Here's how the part is built. I have some questions about the finished solid (model axes, mm). A direction names the side the tool comes from. Round coordinates to 2 decimals unless told otherwise and drop trailing zeros. Order: outer loops, then holes, each group sorted by start corner. A loop starts at its lowest first (then second) coordinate and runs counter-clockwise, first axis right, second up. Notation, with made-up numbers: (-21.5, 78) - (18.5, 78) arc R23 cw to (18.5, 106) - close; hole circle Ø6 at (66.25, 24). An arc over 180 degrees is marked (long way). Answer as a JSON object with one key per item and string values.
```python
from build123d import *

# Parameters (mm, degrees)
SKETCH_1_R          = 35
EXTRUDE_2_DEPTH     = 63.5
SKETCH_3_R          = 2
CUT_EXTRUDE_1_DEPTH = 20


with BuildPart() as part:
    # 草图1 → 凸台-拉伸2 (new body)
    with BuildSketch(Plane.XY):
        Circle(SKETCH_1_R)
    extrude(amount=EXTRUDE_2_DEPTH)

    # 草图3 → 切除-拉伸1 (cut)
    with BuildSketch(Plane.XY.offset(63.5)):
        with Locations((-23, 0)):
            Circle(SKETCH_3_R)
        with Locations((-11.5, 19.918584287)):
            Circle(SKETCH_3_R)
        with Locations((11.5, 19.918584287)):
            Circle(SKETCH_3_R)
        with Locations((23, 0)):
            Circle(SKETCH_3_R)
        with Locations((11.5, -19.918584287)):
            Circle(SKETCH_3_R)
        with Locations((-11.5, -19.918584287)):
            Circle(SKETCH_3_R)
    cut_extrude_1 = extrude(amount=-CUT_EXTRUDE_1_DEPTH, mode=Mode.SUBTRACT)

    # 镜向1: 切除-拉伸1 across plane
    add(cut_extrude_1.mirror(Plane.XY.offset(31.75)), mode=Mode.SUBTRACT)


solid = part.part
```
1. For faces 3 (the face through (-13.087, 18.702, 9.86)), 4 (the face through (-13.087, 18.702, 53.64)), 5 (the face through (0, 0, 63.5)), which set-ups out of +Z, -Z, +X, -X, +Y, -Y let a thin tool reach every point of the face, with its end or its side?
Responses:
{"face 3": "-Z", "face 4": "+Z", "face 5": "+Z, +X, -X, +Y, -Y"}
2. If I drill on L1, parallel to Y at x = -11, z = 48; L2, parallel to X at y = 19, z = 15; L3, parallel to Y at x = 11.5, z = 53, over which ranges is the centre line in solid material (lowest first)? Write a range as [from, to].
Responses:
{"L1": "[-33.23, -21.86], [-17.98, 17.98], [21.86, 33.23]", "L2": "[-29.39, -13.28], [-9.72, 9.72], [13.28, 29.39]", "L3": "[-33.06, -21.92], [-17.92, 17.92], [21.92, 33.06]"}
3. Thinking about a two-plate mould opening in Y: for faces 1 (the face through (9.913, 18.702, 9.86)), 2 (the face through (0, 0, 0)), which applies, pulls with the +Y half, pulls with the -Y half, needs draft (parallel to the pull), parting line crosses it, or undercut?
Responses:
{"face 1": "undercut", "face 2": "needs draft"}
4. Imagine slicing it at D-D (z = 38). List the corners of the cut face in (x, y) for me.
Responses:
{"outline": "circle Ø70 at (0, 0)"}
5. Imagine slicing it at B-B (z = 50.5). List the corners of the cut face in (x, y) for me, plus the area to 3 significant figures.
Responses:
{"outline": "circle Ø70 at (0, 0); hole circle Ø4 at (-23, 0); hole circle Ø4 at (-11.5, -19.92); hole circle Ø4 at (-11.5, 19.92); hole circle Ø4 at (11.5, -19.92); hole circle Ø4 at (11.5, 19.92); hole circle Ø4 at (23, 0)", "area": "3,770 mm2"}
6. Imagine slicing it at A-A (y = 0). List the corners of the cut face in (x, z) for me, plus the area to 4 significant figures.
Responses:
{"outline": "(-35, 0) - (-25, 0) - (-25, 20) - (-21, 20) - (-21, 0) - (21, 0) - (21, 20) - (25, 20) - (25, 0) - (35, 0) - (35, 63.5) - (25, 63.5) - (25, 43.5) - (21, 43.5) - (21, 63.5) - (-21, 63.5) - (-21, 43.5) - (-25, 43.5) - (-25, 63.5) - (-35, 63.5) - close", "area": "4,125 mm2"}
7. For P1, Ø3, axis at x = -23, y = 0, coming from the -Z side; P2, Ø4, axis at x = -12, z = 30.5, coming from the +Y side; P3, Ø1.2, axis at x = 11.5, y = -20, coming from the +Z side, each with a flat end and sliding along its axis, tell me the tip position at first contact or that it passes through.
Responses:
{"P1": "z = 20", "P2": "y = 33.54", "P3": "z = 43.5"}
8. Imagine slicing it at C-C (x = 23). List the corners of the cut face in (y, z) for me, plus the area to 3 significant figures.
Responses:
{"outline": "(-26.38, 0) - (-2, 0) - (-2, 20) - (2, 20) - (2, 0) - (26.38, 0) - (26.38, 63.5) - (2, 63.5) - (2, 43.5) - (-2, 43.5) - (-2, 63.5) - (-26.38, 63.5) - close", "area": "3,190 mm2"}
